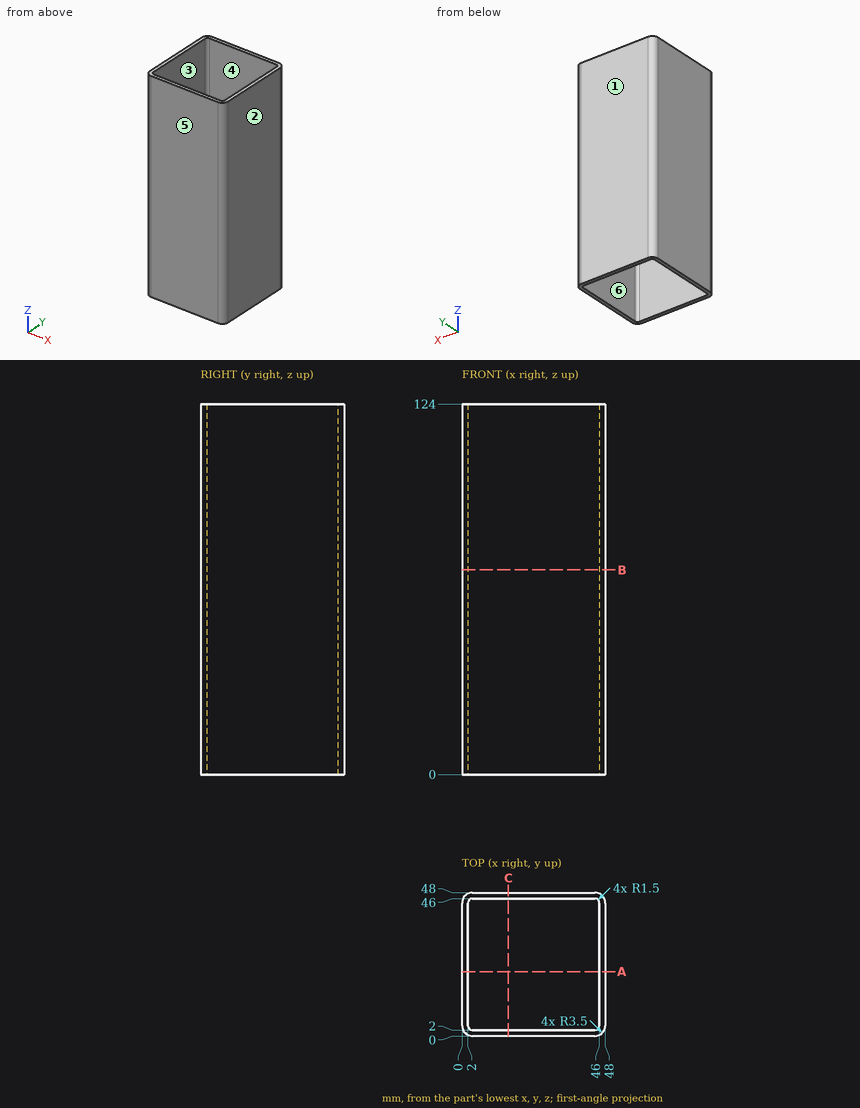
Answer from the drawing. Dimensions are ordinates in mm from the lowest x, y and z of the part. A direction names the side the tool comes from. Round coordinates to 2 decimals unless told otherwise and drop trailing zeros. Write each loop counter-clockwise with the first axis right and the second up, starting at its lowest first coordinate (ties: lowest second). Pieces come first, ordered by that corner, then holes.
1. Determine the mould class of the marked faces 1, 2, 3 and 4 for opening direction X: pulls with the +X half, pulls with the -X half, needs draft (parallel to the pull), parting line crosses it, or undercut.
2. The part is cut by section B-B, the plane z = 68.5. Determine the outline of the cut face in (x, y).
3. Which of the six approach directions +Z, -Z, +X, -X, +Y, -Y give full straight-line access (tool end or side, diameter ignored) to the marked faces 5 and 6?
4. A straight line is drawn through the part: L1, parallel to X at y = 34, z = 84. Find the intervals that lie inside material, in ascending order.
5. The part is cut by section A-A, the plane y = 21.5. Determine the outline of the cut face in (x, z).
Values:
1. face 1: needs draft
1. face 2: pulls with the +X half
1. face 3: undercut
1. face 4: undercut
2. outline: (0, 3.5) arc R3.5 ccw to (3.5, 0) - (44.5, 0) arc R3.5 ccw to (48, 3.5) - (48, 44.5) arc R3.5 ccw to (44.5, 48) - (3.5, 48) arc R3.5 ccw to (0, 44.5) - close; hole (2, 3.5) arc R1.5 ccw to (3.5, 2) - (44.5, 2) arc R1.5 ccw to (46, 3.5) - (46, 44.5) arc R1.5 ccw to (44.5, 46) - (3.5, 46) arc R1.5 ccw to (2, 44.5) - close
3. face 5: +Z, -Z, +X, -X, -Y
3. face 6: +Z, -Z
4. L1: x = 0 to 2, 46 to 48
5. outline: (0, 0) - (2, 0) - (2, 124) - (0, 124) - close; (46, 0) - (48, 0) - (48, 124) - (46, 124) - close
